Read the model definition and answer for the solid it produces. Units are mm, in the model's axes. A direction names the side the tool comes from. Give positions to 0.01 mm unless a question says otherwise; leave off trailing zeros. Loops run counter-clockwise (first coordinate to the right, second up) from the corner with the lowest first, then second, coordinate; pieces in that order, holes last.
(1) Each of these flat-tipped pins is pushed along its axis until it touches: P1, Ø12, axis at x = 44, y = 33.5, coming from the +Z side; P2, Ø12, axis at y = 45, z = -18.5, coming from the +X side; P3, Ø8, axis at x = 48.5, z = -40.5, coming from the +Y side; P4, Ø2, axis at x = 14, z = -53, coming from the +Y side. Where does it stop, or does it pass through?
(2) Find section A-A, the plane x = 0. Write down the section's boundary in (y, z), then the cut area to 3 significant figures.
(3) Find section D-D, the plane x = -16. Write down the section's boundary in (y, z), then the cut area to 3 significant figures.
(4) Find section B-B, the plane z = -35.5. Write down the section's boundary in (x, y).
(5) Which of the six approach directions +Z, -Z, +X, -X, +Y, -Y give full straight-line access (tool end or side, diameter ignored) to faces 5 (the face through (-58, 5, -30)), 6 (the face through (0, 56, -15)), 7 (the face through (0, 30, -30)), 8 (the face through (-50, 10, -30))?
(6) Find section C-C, the plane y = 22. Write down the section's boundary in (x, z).
(7) Determine the mould class of faces 1 (the face through (-22, 45, -30)), 2 (the face through (0, 56, -45)), 3 (the face through (1, 34, -60)), 4 (the face through (50, 10, -30)) for opening direction Z: pulls with the +Z half, pulls with the -Z half, needs draft (parallel to the pull), parting line crosses it, or undercut.
(8) Straight lines are drawn through the part: probe 1 along Y at (x, z) = (0, -51); probe 2 along Z at (x, y) = (13, 50.5); probe 3 along Y at (x, z) = (48, -5). For each, find the intervals that lie inside material, in ascending order.
```python
from build123d import *

# Parameters (mm, degrees)
BOSS_EXTRUDE1_DEPTH = 60
BOSS_EXTRUDE2_DEPTH = 15
SKETCH5_R           = 10
CUT_EXTRUDE1_DEPTH  = 107.5286833


with BuildPart() as part:
    # Sketch1 → Boss-Extrude1 (new body)
    with BuildSketch(Plane.XY):
        Polygon((-58, 0), (-58, 10), (-42, 10), (-30, 45), (30, 45), (42, 10), (58, 10), (58, 0), (25, 0), (9.917302162, 30), (-9.917302162, 30), (-25, 0), align=None)
    extrude(amount=-BOSS_EXTRUDE1_DEPTH)

    # Sketch2 → Boss-Extrude2 (add)
    with BuildSketch(Plane.XY):
        with BuildLine():
            Line((-18.06294145, 33.874117101), (18.06294145, 33.874117101))
            ThreePointArc((18.06294145, 33.874117101), (0, 66.214502683), (-18.06294145, 33.874117101))
        make_face()
    boss_extrude2 = extrude(amount=-BOSS_EXTRUDE2_DEPTH)

    # Sketch5 → Cut-Extrude1 (cut, through all)
    with BuildSketch(Plane.XY):
        with Locations((0, 45)):
            Circle(SKETCH5_R)
    cut_extrude1 = extrude(amount=-CUT_EXTRUDE1_DEPTH, mode=Mode.SUBTRACT)

    # Mirror1: Boss-Extrude2, Cut-Extrude1 across plane
    add(boss_extrude2.mirror(Plane.XY.offset(-30)))
    add(cut_extrude1.mirror(Plane.XY.offset(-30)), mode=Mode.SUBTRACT)


solid = part.part
```
Entries:
1. P1: passes through
1. P2: stops at x = 32.06
1. P3: stops at y = 10
1. P4: stops at y = 61.76
2. outline: (30, -60) - (35, -60) - (35, 0) - (30, 0) - close; (55, -60) - (66.21, -60) - (66.21, -45) - (55, -45) - close; (55, -15) - (66.21, -15) - (66.21, 0) - (55, 0) - close
2. area: 636 mm2
3. outline: (17.9, -60) - (58.93, -60) - (58.93, -45) - (45, -45) - (45, -15) - (58.93, -15) - (58.93, 0) - (17.9, 0) - close
3. area: 2,040 mm2
4. outline: (-58, 0) - (-25, 0) - (-9.92, 30) - (9.92, 30) - (25, 0) - (58, 0) - (58, 10) - (42, 10) - (30, 45) - (10, 45) arc R10 cw to (-10, 45) - (-30, 45) - (-42, 10) - (-58, 10) - close
5. face 5: +Z, -Z, -X, +Y, -Y
5. face 6: +X, -X, +Y
5. face 7: +Z, -Z, -Y
5. face 8: +Z, -Z, -X, +Y
6. outline: (-37.89, -60) - (-13.94, -60) - (-13.94, 0) - (-37.89, 0) - close; (13.94, -60) - (37.89, -60) - (37.89, 0) - (13.94, 0) - close
7. face 1: undercut
7. face 2: undercut
7. face 3: pulls with the -Z half
7. face 4: needs draft
8. probe 1: y = 30 to 35, 55 to 66.21
8. probe 2: z = -60 to -45, -15 to 0
8. probe 3: y = 0 to 10
